from build123d import *

# Parameters (mm, degrees)
BOSS_EXTRUDE1_DEPTH                       = 2.54
CSK_FOR_8_FLAT_HEAD_MACHINE_SCREW_2_COUNT = 2
CSK_FOR_8_FLAT_HEAD_MACHINE_SCREW_2_PITCH = 18.548356757
BOSS_EXTRUDE2_DEPTH                       = 25.4
M7X1_0_TAPPED_HOLE1_D                     = 6
SKETCH6_R                                 = 6.05
BOSS_EXTRUDE3_DEPTH                       = 12.7


with BuildPart() as part:
    # Sketch1 → Boss-Extrude1 (new body)
    # profile 1 of 2: a face of its own
    with BuildSketch(Plane.XY):
        Polygon((6.599113577, -11.43), (13.198227154, 0), (6.599113577, 11.43), (-6.599113577, 11.43), (-13.198227154, 0), (-6.599113577, -11.43), align=None)
        Polygon((-3.666174209, -6.35), (3.666174209, -6.35), (7.332348419, 0), (3.666174209, 6.35), (-3.666174209, 6.35), (-7.332348419, 0), align=None, mode=Mode.SUBTRACT)
    # profile 2 of 2: a face of its own
    with BuildSketch(Plane.XY):
        Polygon((-7.332348419, 0), (-3.666174209, -6.35), (3.666174209, -6.35), (7.332348419, 0), (3.666174209, 6.35), (-3.666174209, 6.35), align=None)
    extrude(amount=BOSS_EXTRUDE1_DEPTH)

    # Sketch3 → CSK for _8 Flat Head Machine Screw _100 (revolve, cut)
    with BuildSketch(Plane(origin=(0, 0, 2.54), x_dir=(0, -1, 0), z_dir=(1, 0, 0))):
        Polygon((0, 0), (0, 2.54), (2.2479, 2.54), (2.2479, 1.651767624), (4.2164, 0), align=None)
    csk_for_8_flat_head_machine_screw_100 = revolve(axis=Axis((0, 0, 8.89), (0, 0, -1)), mode=Mode.SUBTRACT)

    # CSK for _8 Flat Head Machine Screw _ 2: CSK for _8 Flat Head Machine Screw _100 ×2
    with Locations(*[Vector(-0.9274068813992224, 0.37405410883101997, 0) * (i * CSK_FOR_8_FLAT_HEAD_MACHINE_SCREW_2_PITCH) for i in range(1, CSK_FOR_8_FLAT_HEAD_MACHINE_SCREW_2_COUNT)]):
        add(csk_for_8_flat_head_machine_screw_100, mode=Mode.SUBTRACT)

    # Sketch1_4 → Boss-Extrude2 (add)
    with BuildSketch(Plane.XY):
        Polygon((6.599113577, 11.43), (-6.599113577, 11.43), (-13.198227154, 0), (-6.599113577, -11.43), (6.599113577, -11.43), (13.198227154, 0), align=None)
        Polygon((3.666174209, -6.35), (7.332348419, 0), (3.666174209, 6.35), (-3.666174209, 6.35), (-7.332348419, 0), (-3.666174209, -6.35), align=None, mode=Mode.SUBTRACT)
    extrude(amount=BOSS_EXTRUDE2_DEPTH)

    # M7x1.0 Tapped Hole1 (through all)
    with Locations(Plane(origin=(0, 11.43, 0), x_dir=(1, 0, 0), z_dir=(0, 1, 0))):
        with Locations((0, -12.7)):
            Hole(M7X1_0_TAPPED_HOLE1_D / 2)

    # Sketch6 → Boss-Extrude3 (add)
    with BuildSketch(Plane(origin=(0, 0, 0), x_dir=(-1, 0, 0), z_dir=(0, 0, -1))):
        Polygon((-13.198227154, 0), (-6.599113577, -11.43), (6.599113577, -11.43), (13.198227154, 0), (6.599113577, 11.43), (-6.599113577, 11.43), align=None)
        Circle(SKETCH6_R, mode=Mode.SUBTRACT)
    extrude(amount=BOSS_EXTRUDE3_DEPTH)


solid = part.part
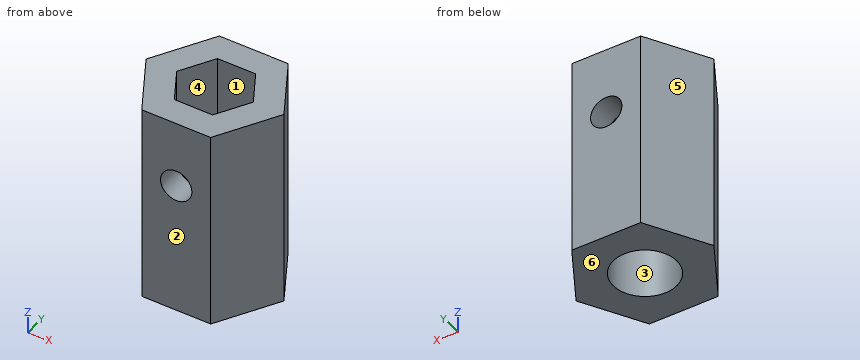
Input: part model. Units: mm. Frame: model coordinates. Face numbers are marked on the shaded views. A direction names the side the tool comes from. Coordinates: 2 decimals unless noted, no trailing zeros. Loops run counter-clockwise (first coordinate to the right, second up) from the corner with the lowest first, then second, coordinate; pieces in that order, holes last. Notation, with made-up numbers: (74, 83) -> (87, 83) arc R18 ccw to (87, 87) -> close; hole circle Ø7 at (8.5, 13). An arc over 180 degrees is marked (long way). Write item = value, one per line. Start each with the question number.
Item 1: Cut plane B-B, the plane x = 0. Return loops of the section in (y, z), plus the area to 3 significant figures.
Item 2: Material intervals for line 1 (X direction, y = 0, z = 0.5); line 2 (Z direction, x = 0, y = 8.35); line 3 (Y direction, x = -5.25, z = -4), sorted ascending.
Item 3: Cut plane D-D, the plane y = 5.5. Return loops of the section in (x, z), plus the area to 3 significant figures.
Item 4: Cut plane C-C, the plane z = -6. Return loops of the section in (x, y).
Item 5: Mould query, pull axis Y, two halves, no side actions, for the marked faces 3, 4, 5 and 6. Classes: pulls with the +Y half, pulls with the -Y half, needs draft (parallel to the pull), parting line crosses it, or undercut.
Item 6: Cut plane A-A, the plane z = 12.7. Return loops of the section in (x, y), plus the area to 3 significant figures.
Item 7: Reachability of the marked faces 1 and 2 from +Z, -Z, +X, -X, +Y, -Y: full face, straight path, thin tool, end or side. Return the list, or none.
Item 8: First-contact query: P1, Ø1.5, axis at y = 8, z = 0, coming from the +X side; P2, Ø1, axis at x = -8, z = 5.5, coming from the -Y side; P3, Ø6, axis at x = -2.5, y = 1.5, coming from the -Z side. Flat tips, straight axial feed; report the tip coordinate or a pass-through.
Ans:
q1.outline = (-11.43, -12.7) -> (-6.05, -12.7) -> (-6.05, 0) -> (-2.25, 0) -> (-2.25, 0.89) -> (-4.22, 2.54) -> (-6.35, 2.54) -> (-6.35, 9.7) -> (-11.43, 9.7) -> close; (-11.43, 15.7) -> (-6.35, 15.7) -> (-6.35, 25.4) -> (-11.43, 25.4) -> close; (2.25, 0) -> (6.05, 0) -> (6.05, -12.7) -> (11.43, -12.7) -> (11.43, 9.7) -> (6.35, 9.7) -> (6.35, 2.54) -> (4.22, 2.54) -> (2.25, 0.89) -> close; (6.35, 15.7) -> (11.43, 15.7) -> (11.43, 25.4) -> (6.35, 25.4) -> close
q1.area = 351 mm²
q2.line_1 = -13.2 to -2.25, 2.25 to 13.2
q2.line_2 = -12.7 to 9.7, 15.7 to 25.4
q2.line_3 = -11.43 to -3.01, 3.01 to 11.43
q3.outline = (-10.02, -12.7) -> (-2.52, -12.7) -> (-2.52, 0) -> (2.52, 0) -> (2.52, -12.7) -> (10.02, -12.7) -> (10.02, 25.4) -> (4.16, 25.4) -> (4.16, 2.54) -> (-4.16, 2.54) -> (-4.16, 25.4) -> (-10.02, 25.4) -> close
q3.area = 510 mm²
q4.outline = (-13.2, 0) -> (-6.6, -11.43) -> (6.6, -11.43) -> (13.2, 0) -> (6.6, 11.43) -> (-6.6, 11.43) -> close; hole circle Ø12.1 at (0, 0)
q5.face_3 = undercut
q5.face_4 = undercut
q5.face_5 = pulls with the +Y half
q5.face_6 = needs draft
q6.outline = (-13.2, 0) -> (-6.6, -11.43) -> (-3, -11.43) -> (-3, -6.35) -> (-3.67, -6.35) -> (-7.33, 0) -> (-3.67, 6.35) -> (-3, 6.35) -> (-3, 11.43) -> (-6.6, 11.43) -> close; (3, -11.43) -> (6.6, -11.43) -> (13.2, 0) -> (6.6, 11.43) -> (3, 11.43) -> (3, 6.35) -> (3.67, 6.35) -> (7.33, 0) -> (3.67, -6.35) -> (3, -6.35) -> close
q6.area = 252 mm²
q7.face_1 = +Z
q7.face_2 = +Z, -Z, +X, -X, -Y
q8.P1 = 9.01
q8.P2 = -9.87
q8.P3 = 0
